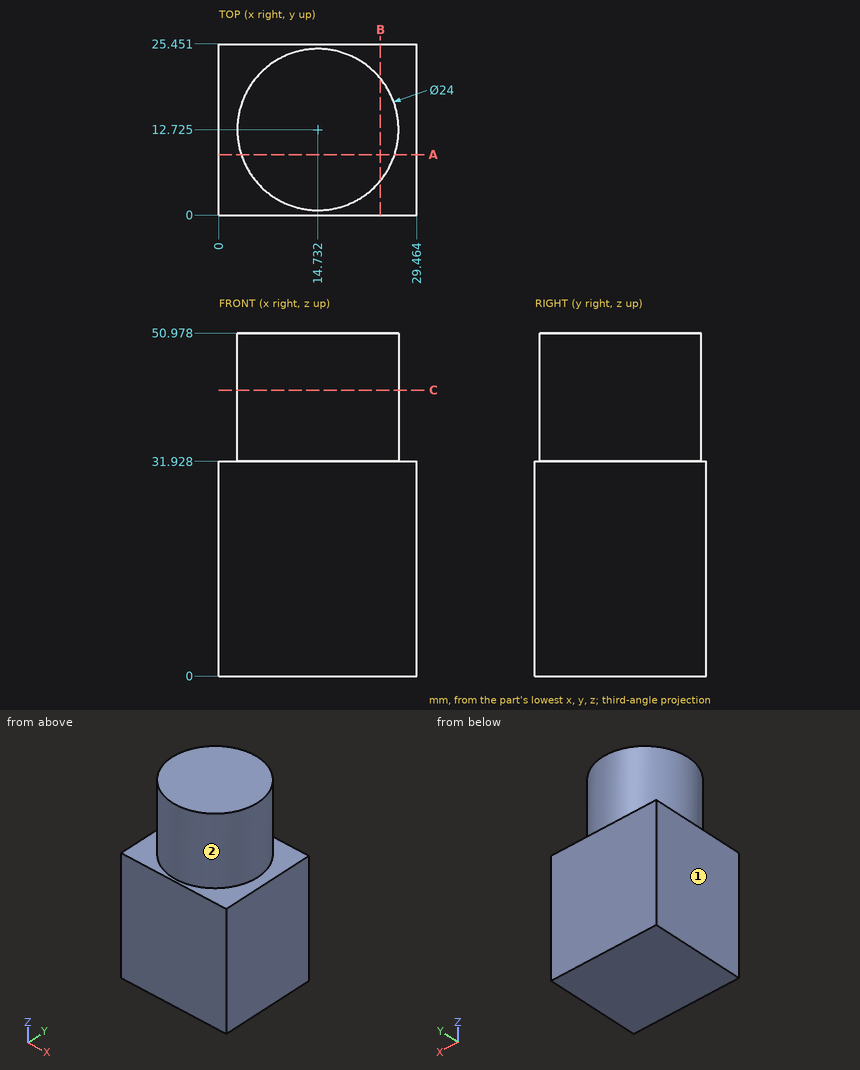
Geometry: see drawing. Coordinates: mm, zero at the bounding-box minimum. A direction names the side the tool comes from. Coordinates: 2 decimals unless noted, no trailing zeros. Order: outer loops, then holes, each group sorted by start corner. A loop starts at its lowest first (then second) coordinate and runs counter-clockwise, first axis right, second up. Notation, with made-up numbers: M 10,-16.75 L 23,-16.75 A22 cw 23,9.25 Z; hole C 66.25,63 d1. An arc over 180 degrees is marked long. Answer as CSV lines item,"result".
1. Material intervals for line 1 (X direction, y = 16, z = 48); line 2 (Y direction, x = 6, z = 46) (1 decimal); line 3 (Z direction, x = 26.5, y = 3), sorted ascending. Write a range as from..to.
Reported:
line 1,"3.19..26.28"
line 2,"4.5..21"
line 3,"0..31.93"
2. Section B-B (x = 24). Return the cut outline in (y, z), then the cut area to 3 significant figures.
Reported:
outline,"M 0,0 L 25.45,0 L 25.45,31.93 L 20.35,31.93 L 20.35,50.98 L 5.1,50.98 L 5.1,31.93 L 0,31.93 Z"
area,"1,100 mm2"
3. Section A-A (y = 9). Return the cut outline in (x, z) (1 decimal).
Reported:
outline,"M 0,0 L 29.5,0 L 29.5,31.9 L 26.1,31.9 L 26.1,51 L 3.3,51 L 3.3,31.9 L 0,31.9 Z"
4. Section C-C (z = 42.5). Return the cut outline in (x, y) (1 decimal), then the cut area to 3 significant figures.
Reported:
outline,"C 14.7,12.7 d24"
area,"452 mm2"
5. Access query for the marked faces 1 and 2. Directions: +Z, -Z, +X, -X, +Y, -Y. A direction counts if a zero-diameter tool reaches every point of the face in a straight line with its end or side. Return the directions, or none.
Reported:
face 1,"+Z, -Z, -X, +Y, -Y"
face 2,"+Z"
6. First-contact query: P1, Ø8, axis at x = 3.5, z = 38.5, coming from the +Y side. Flat tip, straight axial feed; report the tip coordinate or a pass-through.
Reported:
P1,"y = 22.3"
